For this review, take the finished solid that the model builds, in its own axes (mm). A direction names the side the tool comes from. Coordinates: 2 decimals unless noted, no trailing zeros. Loops run counter-clockwise (first coordinate to the right, second up) from the corner with the lowest first, then second, coordinate; pieces in that order, holes last. Notation, with made-up numbers: M 51.25,12 L 87.25,12 A23 cw 87.25,20 Z; hole C 82,52.25 d8. An arc over 180 degrees is marked long. Put each result on its own line as item: value.
```python
from build123d import *

# Parameters (mm, degrees)
ESQUISSE2_R             = 2.85
ESQUISSE2_R_2           = 1
ENL_V_MAT_EXTRU_1_DEPTH = 10
CONG_1_R                = 1
ESQUISSE3_W             = 0.4
ESQUISSE3_H             = 2.2
BOSS_EXTRU_1_DEPTH      = 6.8
ENL_V_MAT_EXTRU_2_REACH = 9.9
ESQUISSE4_R             = 0.6
ENL_V_MAT_EXTRU_3_REACH = 9.9
ESQUISSE6_R             = 0.6


with BuildPart() as part:
    # Esquisse1 → Révolution1 (revolve)
    with BuildSketch(Plane.XY):
        Polygon((0, -6), (-3.75, -6), (-3.75, 1.9), (-5, 1.9), (-5, 5.1), (-4.4, 5.1), (-4.4, 5.35), (-3.75, 6), (0, 6), align=None)
    revolve(axis=Axis((0, 6, 0), (0, -1, 0)))

    # Esquisse2 → Enlèv. mat.-Extru.1 (cut)
    with BuildSketch(Plane(origin=(0, 6, 0), x_dir=(1, 0, 0), z_dir=(0, 1, 0))):
        Circle(ESQUISSE2_R)
        Circle(ESQUISSE2_R_2, mode=Mode.SUBTRACT)
    extrude(amount=-ENL_V_MAT_EXTRU_1_DEPTH, mode=Mode.SUBTRACT)

    # Congé1
    cong_1_edges = [part.edges().sort_by_distance(p)[0] for p in [
        (-1, 6, 0),
    ]]
    fillet(cong_1_edges, radius=CONG_1_R)

    # Esquisse3 → Boss.-Extru.1 (add)
    with BuildSketch(Plane.XZ.offset(6)):
        with Locations((-2.7, 0)):
            Rectangle(ESQUISSE3_W, ESQUISSE3_H)
        with Locations((2.7, 0)):
            Rectangle(ESQUISSE3_W, ESQUISSE3_H)
    extrude(amount=BOSS_EXTRU_1_DEPTH)

    # Esquisse4 → Enlèv. mat.-Extru.2 (cut, up to next)
    with BuildSketch(Plane(origin=(2.9, 0, 0), x_dir=(0, 0, -1), z_dir=(1, 0, 0)), mode=Mode.PRIVATE) as enl_v_mat_extru_2_sk1:
        with BuildLine():
            ThreePointArc((1.1, -9.4), (0, -10.5), (-1.1, -9.4))
            Line((-1.1, -9.4), (-1.1, -12.8))
            Line((-1.1, -12.8), (1.1, -12.8))
            Line((1.1, -12.8), (1.1, -9.4))
        make_face()
    enl_v_mat_extru_2_tool1 = extrude(enl_v_mat_extru_2_sk1.sketch, amount=-ENL_V_MAT_EXTRU_2_REACH, mode=Mode.PRIVATE) & part.part
    add(enl_v_mat_extru_2_tool1.solids().sort_by_distance((2.9, -11.520085, 0))[0], mode=Mode.SUBTRACT)
    # Esquisse4 → Enlèv. mat.-Extru.2 (cut, up to next)
    with BuildSketch(Plane(origin=(2.9, 0, 0), x_dir=(0, 0, -1), z_dir=(1, 0, 0)), mode=Mode.PRIVATE) as enl_v_mat_extru_2_sk2:
        with Locations((0, -9.4)):
            Circle(ESQUISSE4_R)
    enl_v_mat_extru_2_tool2 = extrude(enl_v_mat_extru_2_sk2.sketch, amount=-ENL_V_MAT_EXTRU_2_REACH, mode=Mode.PRIVATE) & part.part
    add(enl_v_mat_extru_2_tool2.solids().sort_by_distance((2.9, -9.4, 0))[0], mode=Mode.SUBTRACT)

    # Esquisse6 → Enlèv. mat.-Extru.3 (cut, up to next)
    with BuildSketch(Plane.ZY.offset(2.9), mode=Mode.PRIVATE) as enl_v_mat_extru_3_sk1:
        with BuildLine():
            ThreePointArc((0, -12.8), (-0.777817459, -12.477817459), (-1.1, -11.7))
            Line((-1.1, -11.7), (-1.1, -12.8))
            Line((-1.1, -12.8), (0, -12.8))
        make_face()
    enl_v_mat_extru_3_tool1 = extrude(enl_v_mat_extru_3_sk1.sketch, amount=-ENL_V_MAT_EXTRU_3_REACH, mode=Mode.PRIVATE) & part.part
    add(enl_v_mat_extru_3_tool1.solids().sort_by_distance((-2.9, -12.554295, -0.854295))[0], mode=Mode.SUBTRACT)
    # Esquisse6 → Enlèv. mat.-Extru.3 (cut, up to next)
    with BuildSketch(Plane.ZY.offset(2.9), mode=Mode.PRIVATE) as enl_v_mat_extru_3_sk2:
        with BuildLine():
            ThreePointArc((1.1, -11.7), (0.777817459, -12.477817459), (0, -12.8))
            Line((0, -12.8), (1.1, -12.8))
            Line((1.1, -12.8), (1.1, -11.7))
        make_face()
    enl_v_mat_extru_3_tool2 = extrude(enl_v_mat_extru_3_sk2.sketch, amount=-ENL_V_MAT_EXTRU_3_REACH, mode=Mode.PRIVATE) & part.part
    add(enl_v_mat_extru_3_tool2.solids().sort_by_distance((-2.9, -12.554295, 0.854295))[0], mode=Mode.SUBTRACT)
    # Esquisse6 → Enlèv. mat.-Extru.3 (cut, up to next)
    with BuildSketch(Plane.ZY.offset(2.9), mode=Mode.PRIVATE) as enl_v_mat_extru_3_sk3:
        with Locations((0, -11.7)):
            Circle(ESQUISSE6_R)
    enl_v_mat_extru_3_tool3 = extrude(enl_v_mat_extru_3_sk3.sketch, amount=-ENL_V_MAT_EXTRU_3_REACH, mode=Mode.PRIVATE) & part.part
    add(enl_v_mat_extru_3_tool3.solids().sort_by_distance((-2.9, -11.7, 0))[0], mode=Mode.SUBTRACT)


solid = part.part
```
(1) Add section B-B (y = 3.5). Write out the cut boundary in (x, z).
Determined:
outline: C 0,0 d10; C 0,0 d2; hole C 0,0 d5.7
(2) Add section D-D (y = -1.5). Write out the cut boundary in (x, z).
Determined:
outline: C 0,0 d7.5; C 0,0 d2; hole C 0,0 d5.7
(3) Wall thickness on line 1 along X through (y, z) = (-1, 0); line 2 along X through (y, z) = (-8, 0.25); line 3 along Y through (x, z) = (2.75, 0): over which ranges is each line inside the solid? List them lowest first. Write a range as [from, to].
Determined:
line 1: x = [-3.75, -2.85], [-1, 1], [2.85, 3.75]
line 2: x = [-2.9, -2.5], [2.5, 2.9]
line 3: y = [-10.5, -10], [-8.8, -4]
(4) Add section C-C (x = 0). Write out the cut boundary in (y, z), plus the area to 3 significant figures.
Determined:
outline: M -6,-3.75 L 1.9,-3.75 L 1.9,-5 L 5.1,-5 L 5.1,-4.4 L 5.35,-4.4 L 6,-3.75 L 6,-2.85 L -4,-2.85 L -4,-1 L 5,-1 A1 ccw 5,1 L -4,1 L -4,2.85 L 6,2.85 L 6,3.75 L 5.35,4.4 L 5.1,4.4 L 5.1,5 L 1.9,5 L 1.9,3.75 L -6,3.75 Z
area: 61.3 mm^2
(5) Tool access review of faces 4 (the flat face through (2.5, -8, 0)), 5 (the flat face through (1, 1.9, -4)), 6 (the cylindrical face through (0, 1, 1)), 7 (the flat face through (-2.9, -9, 0)): name each direction out of +Z, -Z, +X, -X, +Y, -Y from which nothing blocks a thin tool from reaching the whole face with its end or side.
Determined:
face 4: +Z, -Z, -Y
face 5: -Y
face 6: +Y
face 7: +Z, -Z, -X, -Y
(6) Draft analysis for pull direction X (two halves, no side actions). For faces 1 (the cylindrical face through (2.703, -8.805, 0.078)), 2 (the flat face through (-2.5, -9, 0)), 3 (the cylindrical face through (3.746, -1.995, -0.165)), state which applies: +X half, -X half, draft (parallel to the pull), parting line (faces both ways), or undercut.
Determined:
face 1: draft
face 2: undercut
face 3: parting line
(7) For pin 1 (6 mm diameter, centred on y = -8, z = 1.5, fed in from -X); pin 2 (0.7 mm diameter, centred on y = -9, z = 0, fed in from +X); pin 3 (3 mm diameter, centred on x = 3, y = -10, fed in from +Z), all flat-tipped, find the tip position at first contact; note any pin that passes through.
Determined:
pin 1: stops at x = -3.75
pin 2: stops at x = 2.9
pin 3: stops at z = 1.1
(8) Add section A-A (y = -8.25). Write out the cut boundary in (x, z).
Determined:
outline: M -2.9,-1.1 L -2.5,-1.1 L -2.5,1.1 L -2.9,1.1 Z; M 2.5,-1.1 L 2.9,-1.1 L 2.9,1.1 L 2.5,1.1 Z
